Here's how the part is built. I have some questions about the finished solid (model axes, mm). Face numbers are marked on the shaded views. A direction names the side the tool comes from. Coordinates: 2 decimals unless noted, no trailing zeros. Order: outer loops, then holes, each group sorted by start corner. A loop starts at its lowest first (then second) coordinate and runs counter-clockwise, first axis right, second up. Notation, with made-up numbers: (-4, 47) -> (11, 47) arc R17 cw to (11, 74) -> close; hole circle Ø6 at (-16.75, -9). An arc over 180 degrees is marked (long way). One line per item, written item: value. Start each with the question number.
```python
from build123d import *

# Parameters (mm, degrees)
BOX_W             = 19
BOX_H             = 12
BOX_DEPTH         = 2
BOX001_W          = 28
BOX001_H          = 19
BOX001_DEPTH      = 2
CYLINDER_R        = 2
CYLINDER_DEPTH    = 2
BOX002_W          = 8
BOX002_H          = 4
BOX002_DEPTH      = 2
CYLINDER001_R     = 2
CYLINDER001_DEPTH = 2
FILLET_R          = 1


with BuildPart() as part:
    # Box → Box (join)
    with BuildSketch(Plane(origin=(-9.5, -6, 0), x_dir=(1, 0, 0), z_dir=(0, 0, 1))):
        with Locations((9.5, 6)):
            Rectangle(BOX_W, BOX_H)
    extrude(amount=BOX_DEPTH)

    # Box001 → Box001 (join)
    with BuildSketch(Plane(origin=(-9.5, 4, 0), x_dir=(0, 0, 1), z_dir=(0, 1, 0))):
        with Locations((14, 9.5)):
            Rectangle(BOX001_W, BOX001_H)
    extrude(amount=BOX001_DEPTH)

    # Cylinder → Cylinder (cut)
    with BuildSketch(Plane(origin=(-2.5, 0.5, 0), x_dir=(1, 0, 0), z_dir=(0, 0, 1))):
        Circle(CYLINDER_R)
    extrude(amount=CYLINDER_DEPTH, mode=Mode.SUBTRACT)

    # Box002 → Box002 (cut)
    with BuildSketch(Plane(origin=(-10, -1.5, 0), x_dir=(1, 0, 0), z_dir=(0, 0, 1))):
        with Locations((4, 2)):
            Rectangle(BOX002_W, BOX002_H)
    extrude(amount=BOX002_DEPTH, mode=Mode.SUBTRACT)

    # Cylinder001 → Cylinder001 (cut)
    with BuildSketch(Plane(origin=(0, 6, 23.5), x_dir=(1, 0, 0), z_dir=(0, -1, 0))):
        Circle(CYLINDER001_R)
    extrude(amount=CYLINDER001_DEPTH, mode=Mode.SUBTRACT)

    # Fillet
    fillet_edges = [part.edges().sort_by_distance(p)[0] for p in [
        (-9.5, 5, 28),
        (9.5, 5, 28),
        (9.5, -6, 1),
        (-9.5, -6, 1),
    ]]
    fillet(fillet_edges, radius=FILLET_R)


solid = part.part
```
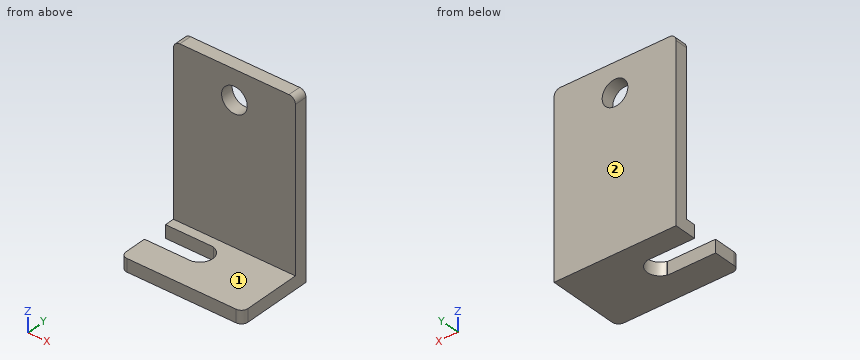
Q1. Imagine slicing it at C-C (y = -4.5). Write out the boundary of the cut face in (x, z), plus the area to 3 significant figures.
Q2. I need wall thicknesses on line 1 (Z direction, x = 0, y = 5.3); line 2 (Y direction, x = 5, z = 11.75); line 3 (Z direction, x = -1.75, y = -4.25). Which ranges of each line are inside material? Lowest first, please.
Q3. Imagine slicing it at D-D (x = 5.5). Write out the boundary of the cut face in (y, z), plus the area to 3 significant figures.
Q4. Imagine slicing it at B-B (z = 23.5). Write out the boundary of the cut face in (x, y).
Q5. For the marked faces 1 and 2, which set-ups out of +Z, -Z, +X, -X, +Y, -Y let a thin tool reach every point of the face, with its end or its side?
Q6. For P1, Ø6.5, axis at x = 0, z = 23.5, coming from the -Y side; P2, Ø2, axis at x = -5.5, y = 2.5, coming from the -Z side, each with a flat end and sliding along its axis, tell me the tip position at first contact or that it passes through.
Q7. Imagine slicing it at A-A (x = 0). Write out the boundary of the cut face in (y, z), plus the area to 3 significant figures.
Completed:
1. outline: (-9.5, 0) -> (9.5, 0) -> (9.5, 2) -> (-9.5, 2) -> close
1. area: 38.0 mm2
2. line 1: z = 0 to 21.5, 25.5 to 28
2. line 2: y = 4 to 6
2. line 3: z = 0 to 2
3. outline: (-6, 0) -> (6, 0) -> (6, 28) -> (4, 28) -> (4, 2) -> (-6, 2) -> close
3. area: 76.0 mm2
4. outline: (-9.5, 4) -> (-2, 4) -> (-2, 6) -> (-9.5, 6) -> close; (2, 4) -> (9.5, 4) -> (9.5, 6) -> (2, 6) -> close
5. face 1: +Z, +X, -X, -Y
5. face 2: +Z, -Z, +X, -X, +Y
6. P1: stops at y = 4
6. P2: stops at z = 0
7. outline: (-6, 0) -> (6, 0) -> (6, 21.5) -> (4, 21.5) -> (4, 2) -> (-6, 2) -> close; (4, 25.5) -> (6, 25.5) -> (6, 28) -> (4, 28) -> close
7. area: 68.0 mm2
